Autodesk Inventor part; units mm, degrees
ref_plane "YZ Plane" through (0, 0, 0) normal (1, 0, 0) x (0, 1, 0)
ref_plane "XZ Plane" through (0, 0, 0) normal (0, 1, 0) x (-1, 0, 0)
ref_plane "XY Plane" through (0, 0, 0) normal (0, 0, 1) x (1, 0, 0)
sketch "Sketch1" plane through (0, 0, 0) normal (0, 0, 1) x (1, 0, 0)
  line L0 (0, 0) -> (0, 15.875)
  line L1 (0, 15.875) -> (0.7937, 15.875)
  line L2 (0.7937, 15.875) -> (0.7938, 0.7937)
  line L3 (0.7938, 0.7937) -> (15.875, 0.7937)
  line L4 (15.875, 0.7937) -> (15.875, 0)
  line L5 (15.875, 0) -> (0, 0)
  dimension "d0" = 15.875
  dimension "d1" = 0.7937
extrude "Extrusion1" add sketch "Sketch1" along normal blind 101.6
sketch "Sketch2" plane through (0.7938, 0.7937, 0) normal (0, 1, 0) x (1, 0, 0)
  line L0 (0, 0) -> (15.0812, 0)
  line L1 (15.0812, -101.6) -> (0, -101.6)
  line L2 (7.5406, 0) -> (7.5406, -101.6) construction
  circle A0 centre (7.5406, -9.525) radius 1.5875
  circle A1 centre (7.5406, -92.075) radius 1.5875
  point P0 (-0.7938, 0)
  dimension "d4" = 9.525
  dimension "d5" = 3.175
  dimension "d6" = 101.6
  dimension "d9" = 82.55
sketch "Sketch3" plane through (0.7938, 0.7937, 0) normal (1, 0, 0) x (0, 0, -1)
  line L0 (0, 15.0812) -> (0, 0)
  line L1 (-101.6, 0) -> (-101.6, 15.0812)
  line L2 (-101.6, 7.5406) -> (0, 7.5406) construction
  circle A0 centre (-9.525, 7.5406) radius 1.5875
  circle A1 centre (-92.075, 7.5406) radius 1.5875
  point P0 (0, -0.7937)
  dimension "d14" = 3.175
  dimension "d15" = 9.525
  dimension "d16" = 101.6
  dimension "d19" = 82.55
extrude "Extrusion2" cut sketch "Sketch2" against normal through all
extrude "Extrusion3" cut sketch "Sketch3" against normal through all
properties part number "Hopper Bracing Front Right P7" material "Aluminum 6061"
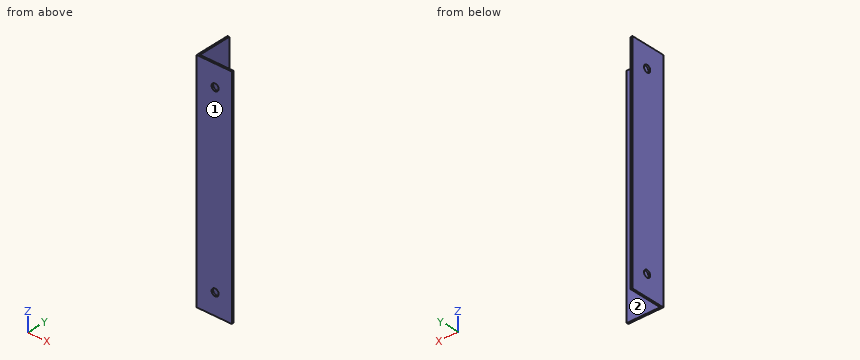
Design review of the part built by this model. Coordinates are the model's own, in mm. Face numbers are marked on the shaded views. A direction names the side the tool comes from. Give positions to 0.01 mm unless a question says otherwise; leave off trailing zeros. Loops run counter-clockwise (first coordinate to the right, second up) from the corner with the lowest first, then second, coordinate; pieces in that order, holes last. Notation, with made-up numbers: (-33.5, -24.5) -> (1.5, -24.5) arc R24 ccw to (1.5, -11.5) -> close; hole circle Ø6 at (21.25, 55.25). An arc over 180 degrees is marked (long way). One line per question, with ' | ' between items. Start each with the question number.
(1) For line 1 (X direction, y = 8.75, z = 65.5), list the stretches that pass through material, from the lowest coordinate up.
(2) We need section B-B (x = 12.5). State the section outline as (y, z) points, and give its area (3 significant figures).
(3) For the marked faces 1 and 2, list the 3-axis set-ups (+Z, -Z, +X, -X, +Y, -Y) from which the entire face can be reached by the end or side of a thin tool; tool diameter is ignored.
(4) We need section A-A (z = 69.5). State the section outline as (x, y) points (3 decimals), and give its area (3 significant figures).
(5) Insertion check: P1, Ø3, axis at x = 3, y = 13.5, coming from the +Z side; P2, Ø5, axis at x = 8.33, z = 9.52, coming from the +Y side; P3, Ø7.5, axis at y = 7, z = 29, coming from the +X side. Each pin has a flat end and moves straight along its axis. Give the tip position at first contact, or say it passes through.
The answers:
1) line 1: x = 0 to 0.79
2) outline: (0, 0) -> (0.79, 0) -> (0.79, 101.6) -> (0, 101.6) -> close | area: 80.6 mm^2
3) face 1: +Z, -Z, +X, -X, -Y | face 2: +Z, -Z, +X, +Y
4) outline: (0, 0) -> (15.875, 0) -> (15.875, 0.794) -> (0.794, 0.794) -> (0.794, 15.875) -> (0, 15.875) -> close | area: 24.6 mm^2
5) P1: passes through | P2: stops at y = 0.79 | P3: stops at x = 0.79
